Verification items for the finished model (mm, model axes). A direction names the side the tool comes from. Coordinates: 2 decimals unless noted, no trailing zeros. Order: outer loops, then holes, each group sorted by start corner. A loop starts at its lowest first (then second) coordinate and runs counter-clockwise, first axis right, second up. Notation, with made-up numbers: (69, 26) -> (90, 26) arc R30 ccw to (90, 65) -> close; hole circle Ø1 at (18.5, -33.75). An arc over 180 degrees is marked (long way). Answer as CSV lines item,"result".
```python
from build123d import *

# Parameters (mm, degrees)
F1_DEPTH    = 4.7625
F2_SIZE2    = 12.7
F2_SIZE     = 3.175
F3_SIZE2    = 12.7
F3_SIZE     = 3.175
F4_R        = 3.175
F5_DEPTH    = 6.35
F6_T4_DEPTH = 35.9361512716
F6_S5_R     = 3.175
F6_T6_DEPTH = 20


# Not quite as in the source:
# - a fillet or chamfer that OpenCascade refuses, or shapes differently, is made with other operations: its cross-section is extruded or revolved along the edge and cut away or added


with BuildPart() as f1:
    # F0 (on Front) → F1 (new body, symmetric)
    with BuildSketch(Plane.XZ):
        with BuildLine():
            ThreePointArc((-38.1, 127), (-36.6107102977, 112.3706344775), (-41.275, 98.425))
            ThreePointArc((-41.275, 98.425), (-20.0980859114, 64.6083576869), (-12.7, 25.4))
            Line((-12.7, 25.4), (-12.7, 0))
            Line((-12.7, 0), (12.7, 0))
            Line((12.7, 0), (12.7, 34.925))
            ThreePointArc((12.7, 34.925), (-0.8424942493, 87.5045721383), (-38.1, 127))
        make_face()
    extrude(amount=F1_DEPTH, both=True)

    # F2
    f2_edges = [f1.edges().sort_by_distance(p)[0] for p in [
        (-0.842494, -4.7625, 87.504572),
        (12.7, -4.7625, 17.4625),
    ]]
    chamfer(f2_edges, length=F2_SIZE, length2=F2_SIZE2)

    # F3
    f3_edges = [f1.edges().sort_by_distance(p)[0] for p in [
        (-0.842494, 4.7625, 87.504572),
    ]]
    f3_side = f1.faces().sort_by_distance((-0.842494, 1.5875, 87.504572))[0]
    chamfer(f3_edges, length=F3_SIZE, length2=F3_SIZE2, reference=f3_side)

    # F4 (on face) → F5 (join)
    with BuildSketch(Plane(origin=(0, 0, 0), x_dir=(1, 0, 0), z_dir=(0, 0, -1))):
        with Locations((-6.35, 0)):
            Circle(F4_R)
        with Locations((3.175, 0)):
            Circle(F4_R)
    extrude(amount=F5_DEPTH)

    # F6: chamfer of 0.508 x 5.08 on 1 edges, made by hand


with BuildPart() as f6_tool2:
    # F6_s3 → F6_t4 (new body)
    with BuildSketch(Plane.XZ.offset(-17.9680756358)):
        Polygon((-12.7, 0.508), (-7.62, 0), (-12.7, 0), align=None)
    extrude(amount=F6_T4_DEPTH)

    # F6_s5 → F6_t6 (cut, symmetric)
    with BuildSketch(Plane.XY.offset(0.3)):
        with Locations((-6.35, 0)):
            Circle(F6_S5_R)
    extrude(amount=F6_T6_DEPTH, both=True, mode=Mode.SUBTRACT)


with BuildPart() as f1_1:
    add(f1.part)

    # F6_t1: cut F6_tool2
    add(f6_tool2.part, mode=Mode.SUBTRACT)


solid = f1_1.part
```
Item 1: Thickness scan on line 1 (X direction, y = -1.5, z = 22.5); line 2 (Z direction, x = -35, y = -0.5); line 3 (X direction, y = -1.5, z = 38). Record the ranges inside material, lowest first.
Answer list:
line 1,"-12.7 to 12.7"
line 2,"90.99 to 124.97"
line 3,"-13.44 to 12.66"
Item 2: Release check for a two-part mould opening along X. For faces 4 (the flat face through (0, -1, 0)), 5 (the flat face through (-16, -4.762, 56)), 6 (the flat face through (6.261, -3.197, 17.218)) record: +X half, -X half, draft (parallel to the pull), parting line (faces both ways), or undercut.
Answer list:
face 4,"undercut"
face 5,"draft"
face 6,"+X half"
Item 3: Tool access check on faces 1 (the flat face through (-12.7, 0, 13)), 2 (the cylindrical face through (-37.086, -0.067, 109.324)), 3 (the cylindrical face through (6.108, 1.216, -3.131)). Record the directions out of +Z, -Z, +X, -X, +Y, -Y that give a thin tool (end or side, any length) a straight path to the whole face; none if there is none.
Answer list:
face 1,"-Z, -X, +Y, -Y"
face 2,"-X, +Y, -Y"
face 3,"-Z"
Item 4: Section check A-A, the plane z = 12. Record the boundary of the cut face in (x, y).
Answer list:
outline,"(-12.7, -4.76) -> (0, -4.76) -> (12.7, -1.59) -> (12.7, 1.59) -> (0, 4.76) -> (-12.7, 4.76) -> close"
Item 5: Depth check by flat-ended pin: pin 1 Ø3 at (y, z) = (-3.5, 15) entering from -X; pin 2 Ø8 at (x, z) = (-4.5, 78.5) entering from +Y; pin 3 Ø3 at (x, z) = (3, 63) entering from -Y. Enter the tip coordinate at first touch or a pass-through.
Answer list:
pin 1,"x = -12.7"
pin 2,"y = 4.43"
pin 3,"y = -3.41"
Item 6: Section check C-C, the plane z = 27. Record the boundary of the cut face in (x, y), plus the area to 3 significant figures.
Answer list:
outline,"(-12.71, -4.76) -> (0, -4.76) -> (12.7, -1.59) -> (12.7, 1.59) -> (0, 4.76) -> (-12.71, 4.76) -> close"
area,"202 mm2"
